```python
from build123d import *

# Parameters (mm, degrees)
F1_DEPTH = 1.27


# Not quite as in the source:
# - a feature of the source that left no trace in its solid (it failed there, or was rolled back) is left out


with BuildPart() as f1:
    # F0 (on Top) → F1 (new body)
    with BuildSketch(Plane.XY):
        Polygon((30.2459372272, 16.8275), (-30.2459372272, 16.8275), (0, -35.56), align=None)
        Polygon((-1.5397931679, -29.591), (1.5397931679, -29.591), (0, -32.258), align=None, mode=Mode.SUBTRACT)
        with BuildLine():
            ThreePointArc((2.38125, -11.8775540145), (0, -20.7645), (-2.38125, -11.8775540145))
            Line((-2.38125, -11.8775540145), (0, -16.002))
            Line((0, -16.002), (2.38125, -11.8775540145))
        make_face(mode=Mode.SUBTRACT)
        with BuildLine():
            Line((-8.7532271537, -1.3180341604), (-12.538315796, -7.874))
            Line((-12.538315796, -7.874), (-4.9681385114, -7.874))
            ThreePointArc((-4.9681385114, -7.874), (-4.6987308277, -7.9855923164), (-4.5871385114, -8.255))
            ThreePointArc((-4.5871385114, -8.255), (-4.6987308277, -8.5244076836), (-4.9681385114, -8.636))
            Line((-4.9681385114, -8.636), (-13.8581385114, -8.636))
            Line((-13.8581385114, -8.636), (-9.4131385114, -0.9370341604))
            ThreePointArc((-9.4131385114, -0.9370341604), (-9.1817928887, -0.7595164205), (-8.8926828325, -0.7975784815))
            ThreePointArc((-8.8926828325, -0.7975784815), (-8.7151650927, -1.0289241042), (-8.7532271537, -1.3180341604))
        make_face(mode=Mode.SUBTRACT)
        with BuildLine():
            Line((-4.9681385114, -7.112), (-11.2184930806, -7.112))
            Line((-11.2184930806, -7.112), (-8.093315796, -1.6990341604))
            ThreePointArc((-8.093315796, -1.6990341604), (-7.5728601171, -1.5595784815), (-7.4334044383, -2.0800341604))
            Line((-7.4334044383, -2.0800341604), (-9.8986703653, -6.35))
            Line((-9.8986703653, -6.35), (-4.9681385114, -6.35))
            ThreePointArc((-4.9681385114, -6.35), (-4.5871385114, -6.731), (-4.9681385114, -7.112))
        make_face(mode=Mode.SUBTRACT)
        with BuildLine():
            ThreePointArc((-10.82675, 2.8605540145), (-17.3324459855, 9.36625), (-8.4455, 6.985))
            Line((-8.4455, 6.985), (-13.208, 6.985))
            Line((-13.208, 6.985), (-10.82675, 2.8605540145))
        make_face(mode=Mode.SUBTRACT)
        with BuildLine():
            Line((4.9681385114, -7.874), (12.538315796, -7.874))
            Line((12.538315796, -7.874), (8.7532271537, -1.3180341604))
            ThreePointArc((8.7532271537, -1.3180341604), (8.7151650927, -1.0289241042), (8.8926828325, -0.7975784815))
            ThreePointArc((8.8926828325, -0.7975784815), (9.1817928887, -0.7595164205), (9.4131385114, -0.9370341604))
            Line((9.4131385114, -0.9370341604), (13.8581385114, -8.636))
            Line((13.8581385114, -8.636), (4.9681385114, -8.636))
            ThreePointArc((4.9681385114, -8.636), (4.6987308277, -8.5244076836), (4.5871385114, -8.255))
            ThreePointArc((4.5871385114, -8.255), (4.6987308277, -7.9855923164), (4.9681385114, -7.874))
        make_face(mode=Mode.SUBTRACT)
        with BuildLine():
            Line((4.9681385114, -6.35), (9.8986703653, -6.35))
            Line((9.8986703653, -6.35), (7.4334044383, -2.0800341604))
            ThreePointArc((7.4334044383, -2.0800341604), (7.5728601171, -1.5595784815), (8.093315796, -1.6990341604))
            Line((8.093315796, -1.6990341604), (11.2184930806, -7.112))
            Line((11.2184930806, -7.112), (4.9681385114, -7.112))
            ThreePointArc((4.9681385114, -7.112), (4.5871385114, -6.731), (4.9681385114, -6.35))
        make_face(mode=Mode.SUBTRACT)
        with BuildLine():
            Line((-3.1251772846, 6.9060341604), (0, 12.319))
            Line((0, 12.319), (3.1251772846, 6.9060341604))
            ThreePointArc((3.1251772846, 6.9060341604), (2.9857216058, 6.3855784815), (2.4652659269, 6.5250341604))
            Line((2.4652659269, 6.5250341604), (0, 10.795))
            Line((0, 10.795), (-2.4652659269, 6.5250341604))
            ThreePointArc((-2.4652659269, 6.5250341604), (-2.9857216058, 6.3855784815), (-3.1251772846, 6.9060341604))
        make_face(mode=Mode.SUBTRACT)
        with BuildLine():
            ThreePointArc((8.4455, 6.985), (17.3324459855, 9.36625), (10.82675, 2.8605540145))
            Line((10.82675, 2.8605540145), (13.208, 6.985))
            Line((13.208, 6.985), (8.4455, 6.985))
        make_face(mode=Mode.SUBTRACT)
        with BuildLine():
            Line((3.7850886423, 7.2870341604), (0, 13.843))
            Line((0, 13.843), (-3.7850886423, 7.2870341604))
            ThreePointArc((-3.7850886423, 7.2870341604), (-4.016434265, 7.1095164205), (-4.3055443212, 7.1475784815))
            ThreePointArc((-4.3055443212, 7.1475784815), (-4.483062061, 7.3789241042), (-4.445, 7.6680341604))
            Line((-4.445, 7.6680341604), (0, 15.367))
            Line((0, 15.367), (4.445, 7.6680341604))
            ThreePointArc((4.445, 7.6680341604), (4.483062061, 7.3789241042), (4.3055443212, 7.1475784815))
            ThreePointArc((4.3055443212, 7.1475784815), (4.016434265, 7.1095164205), (3.7850886423, 7.2870341604))
        make_face(mode=Mode.SUBTRACT)
    extrude(amount=F1_DEPTH)


solid = f1.part
```
The listing builds one solid part. Answer for the finished solid, in the listing's coordinates (mm). Give positions to 0.01 mm unless a question says otherwise; leave off trailing zeros. Loops run counter-clockwise (first coordinate to the right, second up) from the corner with the lowest first, then second, coordinate; pieces in that order, holes last. Notation, with made-up numbers: (-1, 81.5) - (37, 81.5) arc R7 cw to (37, 85.5) - close; hole circle Ø8 at (74.5, -29). An arc over 180 degrees is marked (long way). Return JSON: item names as keys, results as strings. Group by question number.
1. Determine the mould class of faces 1 (the flat face through (-15.335, -9, 0.626)), 2 (the flat face through (8.68, -4.24, 0.63)), 3 (the flat face through (0, 16.828, 1)) for opening direction X: pulls with the +X half, pulls with the -X half, needs draft (parallel to the pull), parting line crosses it, or undercut.
2. Given pin 1 Ø0.6 at (x, z) = (-0.5, 1) entering from -Y, flat-ended and moving along its own axis, determine where the tip first touches the part or whether it passes through.
3. Find section C-C (z = 0.95). State how many separate pieces and enclosed holes the cut face has, then the cut area to 3 significant figures.
4. Find section A-A (x = 17). Write down the section's boundary in (y, z).
5. Find section B-B (y = 5.5). Write down the section's boundary in (x, z).
6. Straight lines are drawn through the part: line 1 (Y direction, x = 8, z = 0.8); line 2 (Y direction, x = -6, z = 1.2); line 3 (Y direction, x = 3, z = 0.8). For each, find the intervals that lie inside material, in ascending order. Write a range as [from, to].
Verdict:
{
 "1": {"face 1": "pulls with the -X half", "face 2": "undercut", "face 3": "needs draft"},
 "2": {"pin 1": "stops at y = -35.21"},
 "3": {"separate pieces": "1", "enclosed holes": "10", "area": "1,340 mm^2"},
 "4": {"outline": "(-6.12, 0) - (4.1, 0) - (4.1, 1.27) - (-6.12, 1.27) - close; (9.87, 0) - (16.83, 0) - (16.83, 1.27) - (9.87, 1.27) - close"},
 "5": {"outline": "(-23.71, 0) - (-17.73, 0) - (-17.73, 1.27) - (-23.71, 1.27) - close; (-12.35, 0) - (12.35, 0) - (12.35, 1.27) - (-12.35, 1.27) - close; (17.73, 0) - (23.71, 0) - (23.71, 1.27) - (17.73, 1.27) - close"},
 "6": {"line 1": "y = [-21.7, -8.64], [-7.87, -7.11], [-6.35, -3.06], [-1.59, 16.83]", "line 2": "y = [-25.17, -8.64], [-7.87, -7.11], [-6.35, 16.83]", "line 3": "y = [-30.36, -19.7], [-12.3, 6.39], [7.12, 8.65], [10.17, 16.83]"}
}
